```python
from build123d import *

# Parameters (mm, degrees)
SKETCH1_W                    = 368.3
SKETCH1_H                    = 469.9
BASE_FLANGE1_DEPTH           = 6.35
EDGE_FLANGE1_STRIP_W         = 26.8732
EDGE_FLANGE1_STRIP_H         = 6.35
EDGE_FLANGE1_STRIP_CUT_DEPTH = 469.9
EDGE_FLANGE1_DEPTH           = 469.9
EDGE_FLANGE2_STRIP_W         = 26.8732
EDGE_FLANGE2_STRIP_H         = 6.35
EDGE_FLANGE2_STRIP_CUT_DEPTH = 469.9
EDGE_FLANGE2_DEPTH           = 469.9
SKETCH14_R                   = 3.429
SKETCH14_W                   = 50.8
SKETCH14_H                   = 254
CUT_EXTRUDE1_DEPTH           = 858.814258741
FILLET1_R                    = 6.35
CUT_EXTRUDE2_DEPTH           = 858.814258741


# Sheet-metal steps are written as plain solids
with BuildPart() as part:
    # Sketch1 → Base-Flange1 (new body)
    with BuildSketch(Plane(origin=(0, 0, 0), x_dir=(1, 0, 0), z_dir=(0, 1, 0))):
        with Locations((184.15, 234.95)):
            Rectangle(SKETCH1_W, SKETCH1_H)
    extrude(amount=BASE_FLANGE1_DEPTH)

    # Edge-Flange1 strip (across the edge) → Edge-Flange1 strip cut (cut)
    with BuildSketch(Plane(origin=(368.3, 6.35, 0), x_dir=(-1, 0, 0), z_dir=(0, 0, -1))):
        with Locations((-6.35, -3.175)):
            Rectangle(EDGE_FLANGE1_STRIP_W, EDGE_FLANGE1_STRIP_H)
    extrude(amount=EDGE_FLANGE1_STRIP_CUT_DEPTH, mode=Mode.SUBTRACT)

    # Edge-Flange1 section (across the edge) → Edge-Flange1 (add)
    with BuildSketch(Plane(origin=(368.3, 6.35, 0), x_dir=(-1, 0, 0), z_dir=(0, 0, -1))):
        with BuildLine():
            Line((0, 0.7366), (0, 609.6))
            Line((0, 609.6), (6.35, 609.6))
            Line((6.35, 609.6), (6.35, 0.7366))
            ThreePointArc((6.35, 0.7366), (6.565745145, 0.215745145), (7.0866, 0))
            Line((7.0866, 0), (7.0866, -6.35))
            ThreePointArc((7.0866, -6.35), (2.075617084, -4.274382916), (0, 0.7366))
        make_face()
    extrude(amount=EDGE_FLANGE1_DEPTH)

    # Edge-Flange2 strip (across the edge) → Edge-Flange2 strip cut (cut)
    with BuildSketch(Plane(origin=(0, 6.35, -469.9), x_dir=(1, 0, 0), z_dir=(0, 0, 1))):
        with Locations((-6.35, -3.175)):
            Rectangle(EDGE_FLANGE2_STRIP_W, EDGE_FLANGE2_STRIP_H)
    extrude(amount=EDGE_FLANGE2_STRIP_CUT_DEPTH, mode=Mode.SUBTRACT)

    # Edge-Flange2 section (across the edge) → Edge-Flange2 (add)
    with BuildSketch(Plane(origin=(0, 6.35, -469.9), x_dir=(1, 0, 0), z_dir=(0, 0, 1))):
        with BuildLine():
            Line((0, 0.7366), (0, 609.6))
            Line((0, 609.6), (6.35, 609.6))
            Line((6.35, 609.6), (6.35, 0.7366))
            ThreePointArc((6.35, 0.7366), (6.565745145, 0.215745145), (7.0866, 0))
            Line((7.0866, 0), (7.0866, -6.35))
            ThreePointArc((7.0866, -6.35), (2.075617084, -4.274382916), (0, 0.7366))
        make_face()
    extrude(amount=EDGE_FLANGE2_DEPTH)

    # Sketch14 → Cut-Extrude1 (cut, through all)
    with BuildSketch(Plane.ZY):
        with Locations(Location((-19.05, 603.25, 0), (0, 0, 270))):
            Circle(SKETCH14_R)
        with Locations(Location((-457.2, 342.9, 0), (0, 0, 270))):
            Circle(SKETCH14_R)
        with Locations(Location((-457.2, 25.4, 0), (0, 0, 270))):
            Circle(SKETCH14_R)
        with Locations((-444.5, 488.95)):
            Rectangle(SKETCH14_W, SKETCH14_H)
    extrude(amount=-CUT_EXTRUDE1_DEPTH, mode=Mode.SUBTRACT)

    # Fillet1
    fillet1_edges = [part.edges().sort_by_distance(p)[0] for p in [
        (365.125, 361.95, -419.1),
        (3.175, 361.95, -419.1),
    ]]
    fillet(fillet1_edges, radius=FILLET1_R)

    # Sketch15 → Cut-Extrude2 (cut, through all)
    with BuildSketch(Plane.ZY):
        with BuildLine():
            ThreePointArc((-421.252860066, 235.717214458), (-247.287179467, 108.52252047), (-37.613208926, 58.729204834))
            ThreePointArc((-37.613208926, 58.729204834), (-23.820795166, 43.963208926), (-38.586791074, 30.170795166))
            ThreePointArc((-38.586791074, 30.170795166), (-259.257504441, 82.575614199), (-442.347139934, 216.441271373))
            ThreePointArc((-442.347139934, 216.441271373), (-441.437971542, 236.62638285), (-421.252860066, 235.717214458))
        make_face()
    extrude(amount=-CUT_EXTRUDE2_DEPTH, mode=Mode.SUBTRACT)


solid = part.part
```
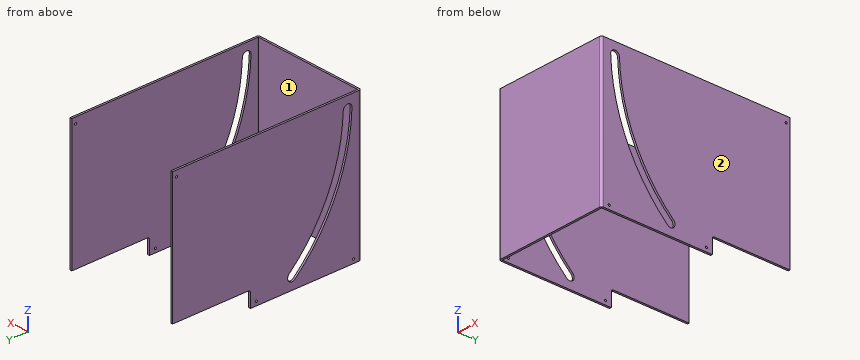
Verification items for the finished model (mm, model axes). Face numbers are marked on the shaded views. A direction names the side the tool comes from. Coordinates: 2 decimals unless noted, no trailing zeros. Write each loop counter-clockwise with the first axis right and the second up, starting at its lowest first coordinate (ties: lowest second). Pieces come first, ordered by that corner, then holes. Notation, with made-up numbers: (38, -27) - (65, -27) arc R15 ccw to (65, -5) - close; hole circle Ø8 at (52, 76). An arc over 180 degrees is marked (long way). Write item = value, one per line.
Q1. Material ranges on L1, parallel to X at y = 231, z = -267; L2, parallel to Y at x = 3, z = -457; L3, parallel to Z at x = 1.75, y = 603.25, recorded low to high. Write a range as from..to.
Answer:
L1 = 0..6.35, 361.95..368.3
L2 = 1.3..21.98, 28.82..339.48, 346.32..361.95
L3 = -419.1..-22.48, -15.62..0
Q2. Go/stop test with flat-tipped pins: pin 1 Ø5 at (x, y) = (4, 431) entering from -Z; pin 2 Ø3 at (x, z) = (3.5, -442) entering from +Y; pin 3 Ø8 at (y, z) = (342.9, -457.2) entering from +X. Record where each tip stops, or that it passes through.
Answer:
pin_1 = -419.1
pin_2 = 361.95
pin_3 = 368.3
Q3. Cross-section at B-B (z = -185). Enter the section's corners in (x, y).
Answer:
outline = (0, 7.09) arc R7.09 ccw to (7.09, 0) - (361.21, 0) arc R7.09 ccw to (368.3, 7.09) - (368.3, 54.38) - (361.95, 54.38) - (361.95, 7.09) arc R0.74 cw to (361.21, 6.35) - (7.09, 6.35) arc R0.74 cw to (6.35, 7.09) - (6.35, 54.38) - (0, 54.38) - close; (0, 84.3) - (6.35, 84.3) - (6.35, 615.95) - (0, 615.95) - close; (361.95, 84.3) - (368.3, 84.3) - (368.3, 615.95) - (361.95, 615.95) - close
Q4. Cross-section at D-D (x = 318.5). Enter the section's corners in (y, z).
Answer:
outline = (0, -469.9) - (6.35, -469.9) - (6.35, 0) - (0, 0) - close
Q5. Cross-section at C-C (y = 146.5). Enter the section's corners in (x, z).
Answer:
outline = (0, -469.9) - (6.35, -469.9) - (6.35, -365.72) - (0, -365.72) - close; (0, -316.08) - (6.35, -316.08) - (6.35, 0) - (0, 0) - close; (361.95, -469.9) - (368.3, -469.9) - (368.3, -365.72) - (361.95, -365.72) - close; (361.95, -316.08) - (368.3, -316.08) - (368.3, 0) - (361.95, 0) - close
Q6. Cross-section at A-A (y = 408). Enter the section's corners in (x, z).
Answer:
outline = (0, -419.1) - (6.35, -419.1) - (6.35, 0) - (0, 0) - close; (361.95, -419.1) - (368.3, -419.1) - (368.3, 0) - (361.95, 0) - close
Q7. Access from +Z, -Z, +X, -X, +Y, -Y to the whole of each face (thin tool, end or side, straight path). Record for the marked faces 1 and 2.
Answer:
face_1 = +Z, -Z, +Y
face_2 = +Z, -Z, +X, +Y, -Y
